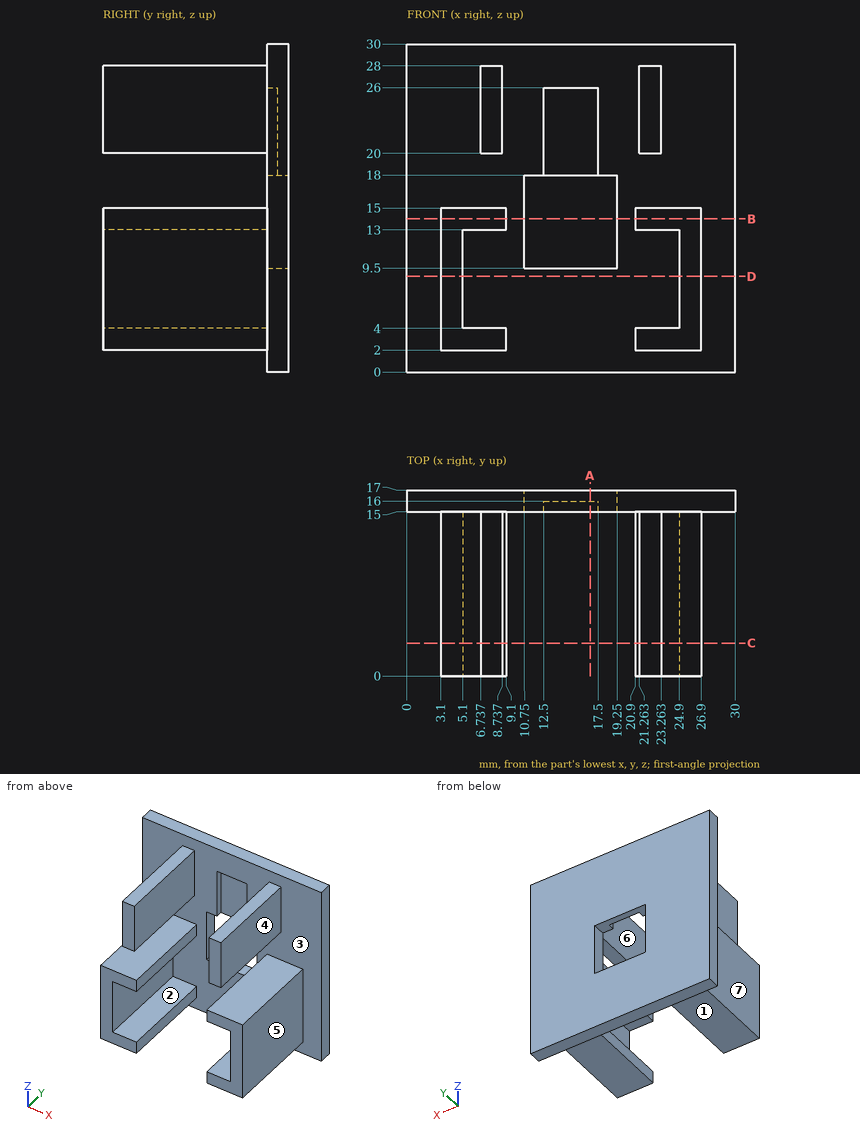
For this review, use the dimensioned drawing (mm, ordinates from the lowest corner) and the shaded views. A direction names the side the tool comes from. Give positions to 0.01 mm unless a question says otherwise; leave off trailing zeros. Order: outer loops, then holes, each group sorted by start corner. A loop starts at its lowest first (then second) coordinate and runs counter-clockwise, first axis right, second up.
1. Add section B-B, the plane z = 14. State the section outline as (x, y) points.
Solution:
outline: (0, 15) - (3.1, 15) - (3.1, 0) - (9.1, 0) - (9.1, 15) - (10.75, 15) - (10.75, 17) - (0, 17) - close; (19.25, 15) - (20.9, 15) - (20.9, 0) - (26.9, 0) - (26.9, 15) - (30, 15) - (30, 17) - (19.25, 17) - close
2. To check wall thickness, follow L1, parallel to Z at x = 21.5, y = 8.25; L2, parallel to X at y = 1.25, z = 7.5; L3, parallel to X at y = 12, z = 3. State the ranges of each line that lie inside material, in increasing order.
Solution:
L1: z = 2 to 4, 13 to 15, 20 to 28
L2: x = 3.1 to 5.1, 24.9 to 26.9
L3: x = 3.1 to 9.1, 20.9 to 26.9
3. Add section A-A, the plane x = 16.75. State the section outline as (y, z) points, then the cut area to 3 significant figures.
Solution:
outline: (15, 0) - (17, 0) - (17, 9.5) - (15, 9.5) - close; (15, 26) - (16, 26) - (16, 18) - (17, 18) - (17, 30) - (15, 30) - close
area: 35.0 mm2
4. Tool access review of the marked faces 5, 6 and 7: name each direction out of +Z, -Z, +X, -X, +Y, -Y from which nothing blocks a thin tool from reaching the whole face with its end or side.
Solution:
face 5: +Z, -Z, +X, -Y
face 6: +Z, -Y
face 7: +Z, -Z, -X, -Y
5. For pin 1 Ø5 at (x, y) = (6, 10.5) entering from +Z; pin 2 Ø0.6 at (y, z) = (5.5, 13.5) entering from +X; pin 3 Ø1.6 at (y, z) = (7, 3) entering from -X; pin 4 Ø1.5 at (y, z) = (9.5, 18) entering from -X, all flat-tipped, find the tip position at first contact; note any pin that passes through.
Solution:
pin 1: stops at z = 28
pin 2: stops at x = 26.9
pin 3: stops at x = 3.1
pin 4: passes through
6. Add section D-D, the plane z = 8.75. State the section outline as (x, y) points, then the cut area to 3 significant figures.
Solution:
outline: (0, 15) - (3.1, 15) - (3.1, 0) - (5.1, 0) - (5.1, 15) - (24.9, 15) - (24.9, 0) - (26.9, 0) - (26.9, 15) - (30, 15) - (30, 17) - (0, 17) - close
area: 120 mm2
7. Mouldability with a two-part tool opening along Z and no side actions: class the marked faces 1, 2, 3 and 4 as +Z half, -Z half, draft (parallel to the pull), parting line (faces both ways), or undercut.
Solution:
face 1: -Z half
face 2: undercut
face 3: undercut
face 4: draft
8. Add section C-C, the plane y = 3. State the section outline as (x, z) points.
Solution:
outline: (3.1, 2) - (9.1, 2) - (9.1, 4) - (5.1, 4) - (5.1, 13) - (9.1, 13) - (9.1, 15) - (3.1, 15) - close; (6.74, 20) - (8.74, 20) - (8.74, 28) - (6.74, 28) - close; (20.9, 2) - (26.9, 2) - (26.9, 15) - (20.9, 15) - (20.9, 13) - (24.9, 13) - (24.9, 4) - (20.9, 4) - close; (21.26, 20) - (23.26, 20) - (23.26, 28) - (21.26, 28) - close
